from build123d import *

# Parameters (mm, degrees)
ESBO_O1_W                                      = 130
ESBO_O1_H                                      = 20
RESSALTO_EXTRUS_O1_DEPTH                       = 95
CORTE_EXTRUS_O2_REACH                          = 22
CORTE_EXTRUS_O3_DEPTH                          = 1
CORTE_EXTRUS_O3_DEPTH_BACK                     = 66
BROCA_DE_ROSQUEAR_DE_CANO_PARA_TARRAXA_D_D     = 6.579997
BROCA_DE_ROSQUEAR_DE_CANO_PARA_TARRAXA_D_DEPTH = 10
BROCA_DE_ROSQUEAR_DE_CANO_PARA_TARRAXA_D_TIP   = 1.976830535
BROCA_DE_ROSQUEAR_DE_CANO_PARA_TARRA_2_D       = 6.579997
BROCA_DE_ROSQUEAR_DE_CANO_PARA_TARRA_2_DEPTH   = 10
BROCA_DE_ROSQUEAR_DE_CANO_PARA_TARRA_2_TIP     = 1.976830535
FILETE2_R                                      = 5
ESBO_O16_W                                     = 50
ESBO_O16_H                                     = 2
CORTE_EXTRUS_O6_DEPTH                          = 40


with BuildPart() as part:
    # Esboço1 → Ressalto-extrusão1 (new body)
    with BuildSketch(Plane.XY):
        Rectangle(ESBO_O1_W, ESBO_O1_H)
    extrude(amount=RESSALTO_EXTRUS_O1_DEPTH)

    # Esboço2 → Corte-extrusão2 (cut, up to next)
    with BuildSketch(Plane(origin=(0, 10, 0), x_dir=(1, 0, 0), z_dir=(0, 1, 0)), mode=Mode.PRIVATE) as corte_extrus_o2_sk1:
        with BuildLine():
            Line((15, 0), (-65, 0))
            Line((-65, 0), (-65, -95))
            Line((-65, -95), (0, -95))
            ThreePointArc((0, -95), (23.934348295, -71.594585279), (35, -40))
            Line((35, -40), (15, 0))
        make_face()
    corte_extrus_o2_tool1 = extrude(corte_extrus_o2_sk1.sketch, amount=-CORTE_EXTRUS_O2_REACH, mode=Mode.PRIVATE) & part.part
    add(corte_extrus_o2_tool1.solids().sort_by_distance((-20.013018, 10, 46.655676))[0], mode=Mode.SUBTRACT)

    # Esboço3 → Corte-extrusão3 (cut, two sides)
    with BuildSketch(Plane(origin=(65, 0, 0), x_dir=(0, 0, -1), z_dir=(1, 0, 0))) as corte_extrus_o3_sk:
        Polygon((200.200134404, 50.040026881), (0, 10), (-95, -9), (-295.200134404, -49.040026881), (-375.280188165, 351.360241926), (120.120080642, 450.440295688), align=None)
    extrude(amount=CORTE_EXTRUS_O3_DEPTH, mode=Mode.SUBTRACT)
    extrude(corte_extrus_o3_sk.sketch, amount=-CORTE_EXTRUS_O3_DEPTH_BACK, mode=Mode.SUBTRACT)

    # Broca de rosquear de cano para tarraxa d
    with Locations(Plane(origin=(65, 0, 0), x_dir=(0, 0, -1), z_dir=(1, 0, 0))):
        with Locations((-20, -1.945)):
            Hole(BROCA_DE_ROSQUEAR_DE_CANO_PARA_TARRAXA_D_D / 2, depth=BROCA_DE_ROSQUEAR_DE_CANO_PARA_TARRAXA_D_DEPTH)
            with Locations((0, 0, -(BROCA_DE_ROSQUEAR_DE_CANO_PARA_TARRAXA_D_DEPTH + BROCA_DE_ROSQUEAR_DE_CANO_PARA_TARRAXA_D_TIP / 2))):  # 118° drill point
                Cone(0, BROCA_DE_ROSQUEAR_DE_CANO_PARA_TARRAXA_D_D / 2, BROCA_DE_ROSQUEAR_DE_CANO_PARA_TARRAXA_D_TIP, mode=Mode.SUBTRACT)

    # Broca de rosquear de cano para tarra 2
    with Locations(Plane(origin=(12, 0, -6), x_dir=(0.447213595, 0, 0.894427191), z_dir=(-0.894427191, 0, 0.447213595))):
        with Locations((26.708203932, -1.945)):
            Hole(BROCA_DE_ROSQUEAR_DE_CANO_PARA_TARRA_2_D / 2, depth=BROCA_DE_ROSQUEAR_DE_CANO_PARA_TARRA_2_DEPTH)
            with Locations((0, 0, -(BROCA_DE_ROSQUEAR_DE_CANO_PARA_TARRA_2_DEPTH + BROCA_DE_ROSQUEAR_DE_CANO_PARA_TARRA_2_TIP / 2))):  # 118° drill point
                Cone(0, BROCA_DE_ROSQUEAR_DE_CANO_PARA_TARRA_2_D / 2, BROCA_DE_ROSQUEAR_DE_CANO_PARA_TARRA_2_TIP, mode=Mode.SUBTRACT)

    # Filete2
    filete2_edges = [part.edges().sort_by_distance(p)[0] for p in [
        (65, -9.5, 95),
    ]]
    fillet(filete2_edges, radius=FILETE2_R)

    # Esboço16 → Corte-extrusão6 (cut)
    with BuildSketch(Plane(origin=(0, 0, 0), x_dir=(-1, 0, 0), z_dir=(0, 0, -1))):
        with Locations((-40, -9)):
            Rectangle(ESBO_O16_W, ESBO_O16_H)
    extrude(amount=-CORTE_EXTRUS_O6_DEPTH, mode=Mode.SUBTRACT)


solid = part.part
Read the model definition and answer for the solid it produces. Units are mm, in the model's axes. A direction names the side the tool comes from. Give positions to 0.01 mm unless a question says otherwise; leave off trailing zeros. Write each loop counter-clockwise with the first axis right and the second up, starting at its lowest first coordinate (ties: lowest second). Pieces come first, ordered by that corner, then holes. Notation, with made-up numbers: (19.25, 35.25) -> (45.25, 35.25) arc R15 cw to (45.25, 58.25) -> close; hole circle Ø5 at (-25, 88.25). An arc over 180 degrees is marked (long way). Answer as a JSON object with one key per item and string values. Group by question number.
1) The mould has two halves that part along X. Classify faces 1 (the flat face through (65, -2, 34)), 2 (the flat face through (46, -10, 73)), 3 (the cylindrical face through (27.08, -0.96, 12.81)): +X half, -X half, draft (parallel to the pull), parting line (faces both ways), or undercut.
2) A tool of negligible diameter and unlimited length cuts with its end or side. For faces 4 (the conical face through (34.094, -1.92, 12.175)), 5 (the flat face through (50, -9, 40)), 6 (the cylindrical face through (27.42, -6.58, 65.49)), from which of +Z, -Z, +X, -X, +Y, -Y can it reach the whole face along a straight path? Write none if from no direction.
3) Consider L1, parallel to Z at x = 20, y = 5.25; L2, parallel to Y at x = 60.5, z = 20 (3 decimals); L3, parallel to X at y = 4.5, z = 16. Determine where each line is inside the solid, lowest interval first. Write a range as from..to.
4) Find section A-A (y = -6.25). Write down the section's boundary in (x, z), and give its area (3 significant figures).
5) Find section C-C (z = 73.5). Write down the section's boundary in (x, y), and give its area (3 significant figures).
6) Each of these flat-tipped pins is pushed along its axis until it touches: P1, Ø1.6, axis at x = 43, y = -9, coming from the -Z side; P2, Ø10.5, axis at y = -1.945, z = 20, coming from the -X side (3 decimals); P3, Ø3, axis at y = -6, z = 75.5, coming from the -X side. Where does it stop, or does it pass through?
7) Find section B-B (x = 9.5). Write down the section's boundary in (y, z), and give its area (3 significant figures).
Values follow:
{
 "1": {"face 1": "+X half", "face 2": "draft", "face 3": "undercut"},
 "2": {"face 4": "none", "face 5": "-Z, +X, -X, -Y", "face 6": "-X, +Y, -Y"},
 "3": {"L1": "z = 0..10", "L2": "y = -8..-5.235, 1.345..6", "L3": "x = 23..65"},
 "4": {"outline": "(15, 0) -> (65, 0) -> (65, 81.25) -> (16.6, 81.25) arc R73.47 cw to (35, 40) -> close", "area": "3,110 mm2"},
 "5": {"outline": "(22.68, -10) -> (65, -10) -> (65, -4.7) -> (22.68, -4.7) -> close", "area": "224 mm2"},
 "6": {"P1": "stops at z = 40", "P2": "stops at x = 22.375", "P3": "stops at x = 20.14"},
 "7": {"outline": "(-10, 88.16) -> (-7.63, 88.16) -> (-9, 95) -> (-10, 95) -> close", "area": "11.5 mm2"}
}
